Verification items for the finished model (mm, model axes). Face numbers are marked on the shaded views. A direction names the side the tool comes from. Round coordinates to 2 decimals unless told otherwise and drop trailing zeros. Write each loop counter-clockwise with the first axis right and the second up, starting at its lowest first coordinate (ties: lowest second). Pieces come first, ordered by that corner, then holes. Notation, with made-up numbers: M -33.5,24 L -19.5,24 A19 cw -19.5,43 Z; hole C -38,-16.5 d10. An arc over 180 degrees is marked long. Answer in a Markdown table with one row per item. Add a question column.
1. Sectioned sample at D-D on z = -9. Record the cut outline in (x, y), plus the area to 3 significant figures.
2. Sectioned sample at B-B on x = 0. Record the cut outline in (y, z), plus the area to 3 significant figures.
3. Set-up check for the marked faces 1 and 2: record each of +Z, -Z, +X, -X, +Y, -Y from which the full face is reachable in a straight line by a thin tool's end or side.
4. Go/stop test with flat-tipped pins: pin 1 Ø5 at (x, y) = (21.5, 10) entering from +Z; pin 2 Ø3 at (x, y) = (33, 6) entering from -Z; pin 3 Ø4 at (x, z) = (17, -28.5) entering from +Y; pin 4 Ø3 at (y, z) = (3, -22) entering from +X. Record where each tip stops, or that it passes through.
5. Sectioned sample at C-C on x = -9.5. Record the cut outline in (y, z), plus the area to 3 significant figures.
6. Sectioned sample at A-A on z = 0. Record the cut outline in (x, y).
7. Material ranges on probe 1 along X at (y, z) = (1.95, 0); probe 2 along X at (y, z) = (10.25, 0), recorded low to high.
```python
from build123d import *

# Parameters (mm, degrees)
SKETCH_1_R          = 43
EXTRUDE_1_DEPTH     = 3
SKETCH_2_R          = 22
SKETCH_2_R_2        = 19
EXTRUDE_2_DEPTH     = 10
SKETCH_3_R          = 19
SKETCH_3_R_2        = 2.320189094
CUT_EXTRUDE_1_DEPTH = 20


with BuildPart() as part:
    # 草图1 → 凸台-拉伸1 (new body)
    with BuildSketch(Plane(origin=(0, 0, 0), x_dir=(1, 0, 0), z_dir=(0, 1, 0))):
        Circle(SKETCH_1_R)
    extrude(amount=EXTRUDE_1_DEPTH)

    # 草图2 → 凸台-拉伸2 (add)
    with BuildSketch(Plane(origin=(0, 3, 0), x_dir=(1, 0, 0), z_dir=(0, 1, 0))):
        Circle(SKETCH_2_R)
        Circle(SKETCH_2_R_2, mode=Mode.SUBTRACT)
    extrude(amount=EXTRUDE_2_DEPTH)

    # 草图3 → 切除-拉伸1 (cut)
    with BuildSketch(Plane(origin=(0, 3, 0), x_dir=(1, 0, 0), z_dir=(0, 1, 0))):
        Circle(SKETCH_3_R)
        with Locations((0, 32.837689205)):
            Circle(SKETCH_3_R_2)
        with Locations((32.837689205, 0)):
            Circle(SKETCH_3_R_2)
        with Locations((0, -32.837689205)):
            Circle(SKETCH_3_R_2)
        with Locations((-32.837689205, 0)):
            Circle(SKETCH_3_R_2)
    extrude(amount=-CUT_EXTRUDE_1_DEPTH, mode=Mode.SUBTRACT)


solid = part.part
```
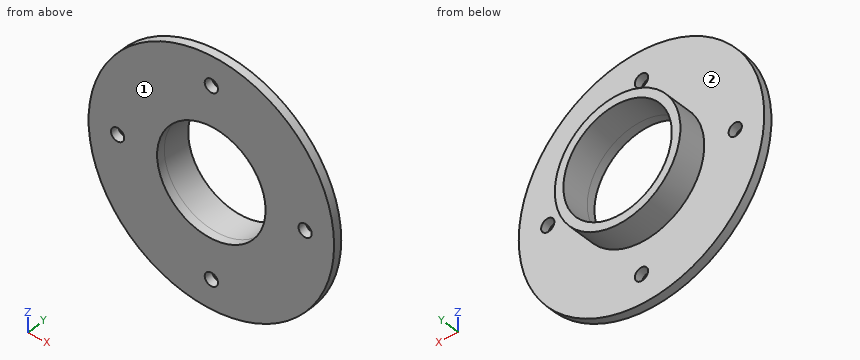
Geometry check:
| question | item | result |
|---|---|---|
| 1 | outline | M -42.05,0 L -16.73,0 L -16.73,13 L -20.07,13 L -20.07,3 L -42.05,3 Z; M 16.73,0 L 42.05,0 L 42.05,3 L 20.07,3 L 20.07,13 L 16.73,13 Z |
| 1 | area | 219 mm2 |
| 2 | outline | M 0,-43 L 3,-43 L 3,-35.16 L 0,-35.16 Z; M 0,-30.52 L 3,-30.52 L 3,-22 L 13,-22 L 13,-19 L 0,-19 Z; M 0,19 L 13,19 L 13,22 L 3,22 L 3,30.52 L 0,30.52 Z; M 0,35.16 L 3,35.16 L 3,43 L 0,43 Z |
| 2 | area | 176 mm2 |
| 3 | face 1 | +Z, -Z, +X, -X, -Y |
| 3 | face 2 | +Y |
| 4 | pin 1 | stops at z = 11.09 |
| 4 | pin 2 | passes through |
| 4 | pin 3 | stops at y = 3 |
| 4 | pin 4 | stops at x = 37.8 |
| 5 | outline | M 0,-41.94 L 3,-41.94 L 3,-19.84 L 13,-19.84 L 13,-16.45 L 0,-16.45 Z; M 0,16.45 L 13,16.45 L 13,19.84 L 3,19.84 L 3,41.94 L 0,41.94 Z |
| 5 | area | 221 mm2 |
| 6 | outline | M -43,0 L -35.16,0 L -35.16,3 L -43,3 Z; M -30.52,0 L -19,0 L -19,13 L -22,13 L -22,3 L -30.52,3 Z; M 19,0 L 30.52,0 L 30.52,3 L 22,3 L 22,13 L 19,13 Z; M 35.16,0 L 43,0 L 43,3 L 35.16,3 Z |
| 7 | probe 1 | x = -43 to -35.16, -30.52 to -19, 19 to 30.52, 35.16 to 43 |
| 7 | probe 2 | x = -22 to -19, 19 to 22 |
